The listing builds one solid part. Answer for the finished solid, in the listing's coordinates (mm). Face numbers are marked on the shaded views. A direction names the side the tool comes from. Round coordinates to 2 decimals unless told otherwise and drop trailing zeros. Write each loop counter-clockwise with the first axis right and the second up, starting at its lowest first coordinate (ties: lowest second). Pieces come first, ordered by that corner, then holes.
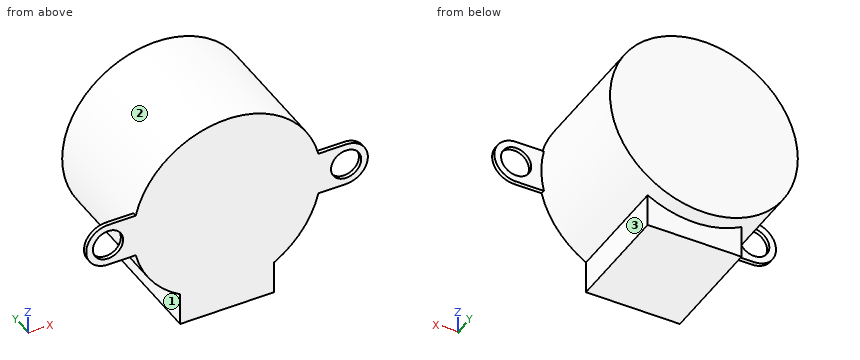
Autodesk Inventor part; units mm, degrees
ref_plane "YZ Plane" through (0, 0, 0) normal (1, 0, 0) x (0, 1, 0)
ref_plane "XZ Plane" through (0, 0, 0) normal (0, 1, 0) x (-1, 0, 0)
ref_plane "XY Plane" through (0, 0, 0) normal (0, 0, 1) x (1, 0, 0)
sketch "Esquisse1" plane through (0, 0, 0) normal (0, 1, 0) x (-1, 0, 0)
  circle A0 centre (0, 0) radius 14
  dimension "d0" = 28
extrude "Extrusion1" add sketch "Esquisse1" along normal blind 19
sketch "Esquisse2" plane through (0, 0, 0) normal (0, -1, 0) x (1, 0, 0)
  line L0 (-21, -3.25) -> (21, -3.25)
  line L1 (21, -3.25) -> (21, 3.25)
  line L2 (21, 3.25) -> (-21, 3.25)
  line L3 (-21, 3.25) -> (-21, -3.25)
  line L4 (-21, -3.25) -> (21, 3.25) construction
  line L5 (21, -3.25) -> (-21, 3.25) construction
  circle A0 centre (-17.75, 0) radius 2.25
  circle A1 centre (17.75, 0) radius 2.25
  arc A2 (-17.75, 3.25) -> (-17.75, -3.25) centre (-17.75, 0) ccw
  arc A3 (17.75, -3.25) -> (17.75, 3.25) centre (17.75, 0) ccw
  circle A4 centre (0, 0) radius 14
  arc A5 (13.6175, -3.25) -> (13.6175, 3.25) centre (0, 0) ccw
  arc A6 (-13.6175, 3.25) -> (-13.6175, -3.25) centre (0, 0) ccw
  line L6 (-17.75, 3.25) -> (-13.6175, 3.25)
  line L7 (-17.75, -3.25) -> (-13.6175, -3.25)
  line L8 (13.6175, -3.25) -> (17.75, -3.25)
  line L9 (17.75, 3.25) -> (13.6175, 3.25)
  dimension "d3" = 42
  dimension "d4" = 6.5
  dimension "d5" = 4.5
  dimension "d6" = 4.5
  dimension "d7" = 3.25
  dimension "d8" = 3.25
extrude "Extrusion2" add sketch "Esquisse2" against normal blind 0.6 contours A2 L2 A4 L0 | A4 L2 A3 L0
sketch "Esquisse3" plane through (0, 0, 0) normal (0, 0, 1) x (1, 0, 0)
  line L0 (7, 0) -> (-7, 0)
  line L1 (-7, 0) -> (-7, 16.5)
  line L2 (-7, 16.5) -> (7, 16.5)
  line L3 (7, 16.5) -> (7, 0)
  point P0 (0, 0)
  dimension "d11" = 16.5
  dimension "d14" = 14
  dimension "d15" = 7
extrude "Extrusion3" add sketch "Esquisse3" against normal blind 17
properties part number "PasAPasCarcasse"
1. Section B-B on x = -6 is taken. Determine the outline of the cut face in (y, z).
Geometry says:
outline: (0, -17) - (16.5, -17) - (16.5, -12.65) - (19, -12.65) - (19, 12.65) - (0, 12.65) - close
2. Section D-D on y = 1.5 is taken. Determine the outline of the cut face in (x, z), plus the area to 3 significant figures.
Geometry says:
outline: (-7, -17) - (7, -17) - (7, -12.12) arc R14 ccw (long way) to (-7, -12.12) - close
area: 666 mm2
3. Straight lines are drawn through the part: line 1 along Z through (x, y) = (-17.75, 0.3); line 2 along X through (y, z) = (13.5, -12.5); line 3 along X through (y, z) = (4, -4). For each, find the intervals that lie inside material, in ascending order.
Geometry says:
line 1: z = -3.25 to -2.25, 2.25 to 3.25
line 2: x = -7 to 7
line 3: x = -13.42 to 13.42
4. Section A-A on y = 17.75 is taken. Determine the outline of the cut face in (x, z).
Geometry says:
outline: circle Ø28 at (0, 0)
5. Given pin 1 (3 mm diameter, centred on y = 16, z = 8, fed in from +X); pin 2 (5 mm diameter, centred on y = 9.5, z = 3, fed in from -X); pin 3 (0.5 mm diameter, centred on x = 16.5, y = 0.5, fed in from +Z), each flat-ended and moving along its own axis, determine where each tip first touches the part or whether it passes through.
Geometry says:
pin 1: stops at x = 12.4
pin 2: stops at x = -13.99
pin 3: stops at z = 3.25
6. Section C-C on z = -8 is taken. Determine the outline of the cut face in (x, y), plus the area to 3 significant figures.
Geometry says:
outline: (-11.49, 0) - (11.49, 0) - (11.49, 19) - (-11.49, 19) - close
area: 437 mm2
7. A tool of negligible diameter and unlimited length cuts with its end or side. For the marked faces 1, 2 and 3, from which of +Z, -Z, +X, -X, +Y, -Y can it reach the whole face along a straight path? Write none if from no direction.
Geometry says:
face 1: -Z, -X, +Y, -Y
face 2: +Y
face 3: -Z, +X, +Y, -Y
